```python
from build123d import *

# Parameters (mm, degrees)
SKETCH1_W                      = 152.4
SKETCH1_H                      = 127
BOSS_EXTRUDE1_DEPTH            = 9.525
F_10_32_TAPPED_HOLE1_D         = 4.0386
F_10_32_TAPPED_HOLE2_OUTLINE_R = 2.0193
F_10_32_TAPPED_HOLE2_DEPTH     = 9.525


# Read off the part's stored shape, not the designer's step: #10-32 Tapped Hole2
with BuildPart() as part:
    # Sketch1 → Boss-Extrude1 (new body)
    with BuildSketch(Plane(origin=(0, 0, 0), x_dir=(1, 0, 0), z_dir=(0, 1, 0))):
        with Locations((76.2, 63.5)):
            Rectangle(SKETCH1_W, SKETCH1_H)
    extrude(amount=BOSS_EXTRUDE1_DEPTH)

    # #10-32 Tapped Hole1 (through all)
    with Locations(Plane(origin=(25.4, 9.525, -6.35), x_dir=(0, 0, 1), z_dir=(0, 1, 0))):
        with Locations((0, 0), (-28.575, 0), (-28.575, 101.6), (0, 101.6)):
            Hole(F_10_32_TAPPED_HOLE1_D / 2)

    # #10-32 Tapped Hole2 outline → #10-32 Tapped Hole2 (cut)
    with BuildSketch(Plane(origin=(0, 0, 0), x_dir=(1, 0, 0), z_dir=(0, 1, 0))):
        with Locations((148.59, 102.87)):
            Circle(F_10_32_TAPPED_HOLE2_OUTLINE_R)
        with Locations((3.81, 102.87)):
            Circle(F_10_32_TAPPED_HOLE2_OUTLINE_R)
    extrude(amount=F_10_32_TAPPED_HOLE2_DEPTH, mode=Mode.SUBTRACT)


solid = part.part
```
CAD build for the part. Positions are in the model's coordinates, mm. Round coordinates to 2 decimals unless told otherwise and drop trailing zeros. Write each loop counter-clockwise with the first axis right and the second up, starting at its lowest first coordinate (ties: lowest second). Pieces come first, ordered by that corner, then holes. Notation, with made-up numbers: (2.5, 39) - (41.5, 39) arc R16 ccw to (41.5, 62) - close; hole circle Ø5 at (75, 38.25). An arc over 180 degrees is marked (long way). Return JSON: item names as keys, results as strings. Group by question number.
Item 1: Band-saw the part on A-A on z = -102.87. List the corners of the cut face in (x, y) (3 decimals), plus the area to 3 significant figures.
Item 2: Band-saw the part on C-C on x = 25.4. List the corners of the cut face in (y, z) (3 decimals), plus the area to 3 significant figures.
Item 3: Probe probe 1 along X at (y, z) = (4, -6.35); probe 2 along X at (y, z) = (3, -36); probe 3 along Z at (x, y) = (3.81, 6). List the from-to ranges inside material, lowest first.
Item 4: Band-saw the part on B-B on x = 148.59. List the corners of the cut face in (y, z) (3 decimals), plus the area to 3 significant figures.
Item 5: Mould opens along X. For faces 1 (the face through (3.547, 4.696, -104.872)), 2 (the face through (125.21, 4.7, -35.86)), 3 (the face through (75, 5, -127)), 4 (the face through (0, 5, -63)) say: +X half, -X half, draft (parallel to the pull), parting line (faces both ways), or undercut.
Item 6: Flat gauge pin, fed straight in: pin 1 Ø2.5 at (x, z) = (148.59, -102.87) entering from +Y. Where does the tip first touch, or does it go through?
Resolved:
{
 "1": {"outline": "(0, 0) - (1.791, 0) - (1.791, 9.525) - (0, 9.525) - close; (5.829, 0) - (146.571, 0) - (146.571, 9.525) - (5.829, 9.525) - close; (150.609, 0) - (152.4, 0) - (152.4, 9.525) - (150.609, 9.525) - close", "area": "1,370 mm²"},
 "2": {"outline": "(0, -127) - (9.525, -127) - (9.525, -36.944) - (0, -36.944) - close; (0, -32.906) - (9.525, -32.906) - (9.525, -8.369) - (0, -8.369) - close; (0, -4.331) - (9.525, -4.331) - (9.525, 0) - (0, 0) - close", "area": "1,130 mm²"},
 "3": {"probe 1": "x = 0 to 23.38, 27.42 to 124.98, 129.02 to 152.4", "probe 2": "x = 0 to 23.69, 27.11 to 125.29, 128.71 to 152.4", "probe 3": "z = -127 to -104.89, -100.85 to 0"},
 "4": {"outline": "(0, -127) - (9.525, -127) - (9.525, -104.889) - (0, -104.889) - close; (0, -100.851) - (9.525, -100.851) - (9.525, 0) - (0, 0) - close", "area": "1,170 mm²"},
 "5": {"face 1": "undercut", "face 2": "undercut", "face 3": "draft", "face 4": "-X half"},
 "6": {"pin 1": "passes through"}
}
